Verification items for the finished model (mm, model axes). Face numbers are marked on the shaded views. Give positions to 0.01 mm unless a question says otherwise; leave off trailing zeros. Loops run counter-clockwise (first coordinate to the right, second up) from the corner with the lowest first, then second, coordinate; pieces in that order, holes last. Notation, with made-up numbers: (8, 35.25) -> (26, 35.25) arc R26 cw to (26, 68.25) -> close; hole circle Ø9 at (89, -32). An arc over 180 degrees is marked (long way). Answer in a Markdown table with one row per item. Add a question column.
Q1. Material ranges on probe 1 along Y at (x, z) = (1, 0); probe 2 along X at (y, z) = (10.75, 0); probe 3 along Y at (x, z) = (-0.4, 0), recorded low to high.
Q2. Release check for a two-part mould opening along X. For the marked faces 1, 2 and 3 record: pulls with the +X half, pulls with the -X half, needs draft (parallel to the pull), parting line crosses it, or undercut.
Q3. Gauge pin test, flat end, axial feed: P1, Ø1.6, axis at x = 0, z = 0, coming from the +Y side. Record the tip position at first contact, or that the pin passes through.
Q4. Section check B-B on x = 0. Enter the section's corners in (y, z).
Q5. Section check D-D on y = 5.75. Enter the section's corners in (x, z).
Q6. Section check C-C on y = 8.75. Enter the section's corners in (x, z), and give its area (3 significant figures).
Q7. Section check A-A on z = 0. Enter the section's corners in (x, y).
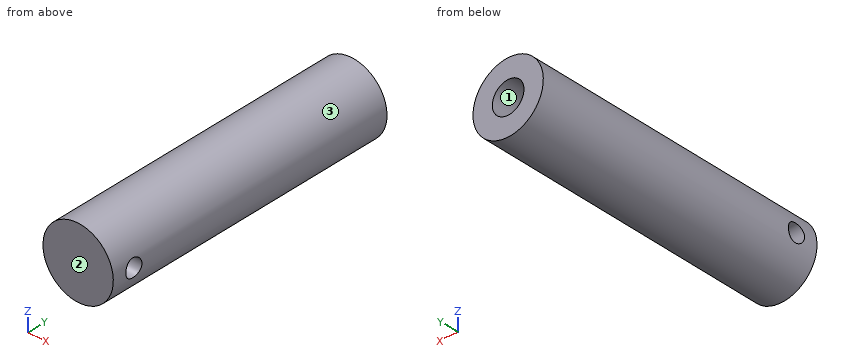
```python
from build123d import *

# Parameters (mm, degrees)
SZKIC1_R                        = 2
DODANIE_WYCI_GNI_CIE1_DEPTH     = 16.9
SZKIC2_R                        = 0.9
WYTNIJ_WYCI_GNI_CIE1_DEPTH      = 10
WYTNIJ_WYCI_GNI_CIE2_DEPTH      = 18.135051794
WYTNIJ_WYCI_GNI_CIE2_DEPTH_BACK = 18.135051794
SZKIC3_R                        = 0.5


with BuildPart() as part:
    # Szkic1 → Dodanie-wyciągnięcie1 (new body)
    with BuildSketch(Plane(origin=(0, 0, 0), x_dir=(1, 0, 0), z_dir=(0, 1, 0))):
        with Locations(Location((0, 0, 0), (0, 0, 270))):
            Circle(SZKIC1_R)
    extrude(amount=DODANIE_WYCI_GNI_CIE1_DEPTH)

    # Szkic2 → Wytnij-wyciągnięcie1 (cut)
    with BuildSketch(Plane(origin=(0, 16.9, 0), x_dir=(1, 0, 0), z_dir=(0, 1, 0))):
        with Locations(Location((0, 0, 0), (0, 0, 270))):
            Circle(SZKIC2_R)
    extrude(amount=-WYTNIJ_WYCI_GNI_CIE1_DEPTH, mode=Mode.SUBTRACT)

    # Szkic3 → Wytnij-wyciągnięcie2 (cut, two sides: drawn at the far end of the back side and taken through both)
    with BuildSketch(Plane(origin=(0, 0, 0), x_dir=(0, 0, -1), z_dir=(1, 0, 0)).offset(-WYTNIJ_WYCI_GNI_CIE2_DEPTH_BACK)):
        with Locations((0, 1.268865349)):
            Circle(SZKIC3_R)
    extrude(amount=WYTNIJ_WYCI_GNI_CIE2_DEPTH + WYTNIJ_WYCI_GNI_CIE2_DEPTH_BACK, mode=Mode.SUBTRACT)


solid = part.part
```
Taken from the geometry:
| question | item | result |
|---|---|---|
| 1 | probe 1 | y = 0 to 0.77, 1.77 to 16.9 |
| 1 | probe 2 | x = -2 to -0.9, 0.9 to 2 |
| 1 | probe 3 | y = 0 to 0.77, 1.77 to 6.9 |
| 2 | face 1 | undercut |
| 2 | face 2 | needs draft |
| 2 | face 3 | parting line crosses it |
| 3 | P1 | stops at y = 6.9 |
| 4 | outline | (0, -2) -> (16.9, -2) -> (16.9, -0.9) -> (6.9, -0.9) -> (6.9, 0.9) -> (16.9, 0.9) -> (16.9, 2) -> (0, 2) -> close; hole circle Ø1 at (1.27, 0) |
| 5 | outline | circle Ø4 at (0, 0) |
| 6 | outline | circle Ø4 at (0, 0); hole circle Ø1.8 at (0, 0) |
| 6 | area | 10.0 mm² |
| 7 | outline | (-2, 0) -> (2, 0) -> (2, 0.77) -> (-2, 0.77) -> close; (-2, 1.77) -> (2, 1.77) -> (2, 16.9) -> (0.9, 16.9) -> (0.9, 6.9) -> (-0.9, 6.9) -> (-0.9, 16.9) -> (-2, 16.9) -> close |
